Could you check a few things on this model? Use its own coordinates, in mm. Round coordinates to 2 decimals unless told otherwise and drop trailing zeros. Loops run counter-clockwise (first coordinate to the right, second up) from the corner with the lowest first, then second, coordinate; pieces in that order, holes last.
from build123d import *

# Parameters (mm, degrees)
F1_DEPTH = 8
F2_W     = 20.4098413018
F2_H     = 2.387965478
F3_DEPTH = 13.1
F4_R     = 0.66
F5_SIZE  = 0.66


with BuildPart() as f1:
    # F0 (on Front) → F1 (new body)
    with BuildSketch(Plane.XZ):
        with BuildLine():
            Line((13.435, 0), (10.445, 0))
            ThreePointArc((10.445, 0), (0, -10.445), (-10.445, 0))
            Line((-10.445, 0), (-13.435, 0))
            ThreePointArc((-13.435, 0), (-10.1247178165, -8.8311558777), (-1.8251281523, -13.3104519919))
            Line((-1.8251281523, -13.3104519919), (1.8251281523, -13.3104519919))
            ThreePointArc((1.8251281523, -13.3104519919), (10.1247178165, -8.8311558777), (13.435, 0))
        make_face()
        with BuildLine():
            ThreePointArc((-10.445, 0), (0, 10.445), (10.445, 0))
            Line((10.445, 0), (13.435, 0))
            ThreePointArc((13.435, 0), (10.1247178165, 8.8311558777), (1.8251281523, 13.3104519919))
            Line((1.8251281523, 13.3104519919), (-1.8251281523, 13.3104519919))
            ThreePointArc((-1.8251281523, 13.3104519919), (-10.1247178165, 8.8311558777), (-13.435, 0))
            Line((-13.435, 0), (-10.445, 0))
        make_face()
        with BuildLine():
            ThreePointArc((1.8251281523, 13.3104519919), (10.1247178165, 8.8311558777), (13.435, 0))
            Line((13.435, 0), (13.4794265032, 13.3104519919))
            Line((13.4794265032, 13.3104519919), (1.8251281523, 13.3104519919))
        make_face()
        with BuildLine():
            Line((-13.4794265032, 13.3104519919), (-13.435, 0))
            ThreePointArc((-13.435, 0), (-10.1247178165, 8.8311558777), (-1.8251281523, 13.3104519919))
            Line((-1.8251281523, 13.3104519919), (-13.4794265032, 13.3104519919))
        make_face()
        with BuildLine():
            ThreePointArc((-1.8251281523, -13.3104519919), (0, -13.435), (1.8251281523, -13.3104519919))
            Line((1.8251281523, -13.3104519919), (-1.8251281523, -13.3104519919))
        make_face()
        with BuildLine():
            Line((-1.8251281523, 13.3104519919), (1.8251281523, 13.3104519919))
            ThreePointArc((1.8251281523, 13.3104519919), (0.9768871079, 13.3994371739), (0.1247091036, 13.4344211874))
            ThreePointArc((0.1247091036, 13.4344211874), (2e-08, 13.435), (-0.1247090636, 13.4344211877))
            ThreePointArc((-0.1247090636, 13.4344211877), (-0.9768870879, 13.3994371754), (-1.8251281523, 13.3104519919))
        make_face()
        with BuildLine():
            ThreePointArc((0.1247091036, 13.4344211874), (0.9768871079, 13.3994371739), (1.8251281523, 13.3104519919))
            Line((1.8251281523, 13.3104519919), (13.4794265032, 13.3104519919))
            Line((13.4794265032, 13.3104519919), (0.1247091036, 13.4344211874))
        make_face()
        with BuildLine():
            Line((-13.4794265032, 13.3104519919), (-1.8251281523, 13.3104519919))
            ThreePointArc((-1.8251281523, 13.3104519919), (-0.9768870879, 13.3994371754), (-0.1247090636, 13.4344211877))
            Line((-0.1247090636, 13.4344211877), (-13.4794265032, 13.3104519919))
        make_face()
        with BuildLine():
            ThreePointArc((-0.1247090636, 13.4344211877), (2e-08, 13.435), (0.1247091036, 13.4344211874))
            Line((0.1247091036, 13.4344211874), (0, 13.4355788373))
            Line((0, 13.4355788373), (-0.1247090636, 13.4344211877))
        make_face()
    extrude(amount=F1_DEPTH)

    # F2 (on face) → F3 (cut)
    with BuildSketch(Plane(origin=(-0.12470907, 0, 13.4344211877), x_dir=(0.9999569176, 0, 0.0092824019), z_dir=(-0.0092824019, 0, 0.9999569176))):
        with Locations((0.124714443, -4)):
            Rectangle(F2_W, F2_H)
    extrude(amount=-F3_DEPTH, mode=Mode.SUBTRACT)

    # F4
    f4_edges = [f1.edges().sort_by_distance(p)[0] for p in [
        (-13.479427, -4, 13.310452),
        (13.479427, -4, 13.310452),
    ]]
    fillet(f4_edges, radius=F4_R)

    # F5
    f5_edges = [f1.edges().sort_by_distance(p)[0] for p in [
        (10.445, 0, 0),
        (10.445, -8, 0),
    ]]
    chamfer(f5_edges, length=F5_SIZE)


solid = f1.part
Item 1: If we section it at A-A, the plane y = -4.75: Please give me the cut outline in (x, z) (3 decimals), then the cut area to 3 significant figures.
Results list:
outline: (-13.477, 12.654) - (-13.435, 0) arc R13.435 ccw to (13.435, 0) - (13.477, 12.654) arc R0.66 ccw to (12.823, 13.317) - (10.206, 13.341) - (10.315, 1.644) arc R10.445 cw (long way) to (-10.105, 2.643) - (-10.204, 13.341) - (-12.823, 13.317) arc R0.66 ccw to start
area: 198 mm2
Item 2: We'd pull the mould along Z, two halves only. Please class faces 1 (the flat face through (3, 0, 11)), 2 (the cylindrical face through (2.264, -3.953, -10.197)): released by +Z, released by -Z, zero draft, split by the parting line, or undercut.
Results list:
face 1: zero draft
face 2: undercut
Item 3: If we section it at B-B, the plane x = 3.75: Count the separate pieces of the cut face and the enclosed holes in it, then the cut area to 3 significant figures.
Results list:
separate pieces: 3
enclosed holes: 0
area: 44.8 mm2
Item 4: Will this pin go through, and if not, where does the flat tip stop? pin 1 (1 mm diameter, centred on x = 1.5, y = -3, fed in from +Z).
Results list:
pin 1: stops at z = 13.43
Item 5: If I drill on line 1 along Z through (x, y) = (-0.25, -7); line 2 along X through (y, z) = (-1.75, 5.75); line 3 along Z through (x, y) = (-2.5, -6.25), over which ranges is the centre line in solid material (lowest first)?
Results list:
line 1: z = -13.43 to -10.44, 10.44 to 13.43
line 2: x = -13.45 to -8.72, 8.72 to 13.45
line 3: z = -13.2 to -10.14, 10.14 to 13.41
Item 6: If we section it at C-C, the plane z = -11.5: Please give me the cut outline in (x, y), then the cut area to 3 significant figures.
Results list:
outline: (-6.95, -8) - (6.95, -8) - (6.95, 0) - (-6.95, 0) - close
area: 111 mm2
